Design review of the part built by this model. Coordinates are the model's own, in mm. Give positions to 0.01 mm unless a question says otherwise; leave off trailing zeros. Order: outer loops, then holes, each group sorted by start corner. A loop starts at its lowest first (then second) coordinate and runs counter-clockwise, first axis right, second up.
```python
from build123d import *

# Parameters (mm, degrees)
F0_W           = 127
F0_H           = 76.2
F1_DEPTH       = 3.175
F3_D           = 5.5
F3_CSINK_D     = 11.2
F3_CSINK_ANGLE = 90
F5_D           = 5.5
F5_CSINK_D     = 11.2
F5_CSINK_ANGLE = 90
F6_R           = 6.35


with BuildPart() as f1:
    # F0 (on Top) → F1 (new body)
    with BuildSketch(Plane.XY):
        Rectangle(F0_W, F0_H)
    extrude(amount=-F1_DEPTH)

    # F3 (through all)
    with Locations(Plane.XY):
        with Locations((-50.8, -25.4), (-50.8, 25.4), (50.8, 25.4), (50.8, -25.4)):
            CounterSinkHole(F3_D / 2, F3_CSINK_D / 2, counter_sink_angle=F3_CSINK_ANGLE)

    # F5 (through all)
    with Locations(Plane(origin=(0, 0, -3.175), x_dir=(1, 0, 0), z_dir=(0, 0, -1))):
        with Locations((0, 0)):
            CounterSinkHole(F5_D / 2, F5_CSINK_D / 2, counter_sink_angle=F5_CSINK_ANGLE)

    # F6
    f6_edges = [f1.edges().sort_by_distance(p)[0] for p in [
        (63.5, -38.1, -1.5875),
        (63.5, 38.1, -1.5875),
        (-63.5, -38.1, -1.5875),
        (-63.5, 38.1, -1.5875),
    ]]
    fillet(f6_edges, radius=F6_R)


solid = f1.part
```
1. For pin 1 (7 mm diameter, centred on x = 50.8, y = 25.4, fed in from -Z) (3 decimals); pin 2 (7 mm diameter, centred on x = 0, y = 0, fed in from -Z) (3 decimals); pin 3 (3.5 mm diameter, centred on x = -50.8, y = -25.4, fed in from +Z); pin 4 (6.5 mm diameter, centred on x = -50.8, y = 25.4, fed in from +Z), all flat-tipped, find the tip position at first contact; note any pin that passes through.
Recorded:
pin 1: stops at z = -3.175
pin 2: stops at z = -1.075
pin 3: passes through
pin 4: stops at z = -2.35
2. Take a section at C-C (z = -1.7). State the section outline as (x, y) points (3 decimals), then the cut area to 3 significant figures.
Recorded:
outline: (-63.5, -31.75) arc R6.35 ccw to (-57.15, -38.1) - (57.15, -38.1) arc R6.35 ccw to (63.5, -31.75) - (63.5, 31.75) arc R6.35 ccw to (57.15, 38.1) - (-57.15, 38.1) arc R6.35 ccw to (-63.5, 31.75) - close; hole circle Ø7.8 at (-50.8, -25.4); hole circle Ø7.8 at (-50.8, 25.4); hole circle Ø8.25 at (0, 0); hole circle Ø7.8 at (50.8, -25.4); hole circle Ø7.8 at (50.8, 25.4)
area: 9,400 mm2
3. Take a section at B-B (y = 25.4). State the section outline as (x, z) points (3 decimals), then the cut area to 3 significant figures.
Recorded:
outline: (-63.5, -3.175) - (-53.55, -3.175) - (-53.55, -2.85) - (-56.4, 0) - (-63.5, 0) - close; (-48.05, -3.175) - (48.05, -3.175) - (48.05, -2.85) - (45.2, 0) - (-45.2, 0) - (-48.05, -2.85) - close; (53.55, -3.175) - (63.5, -3.175) - (63.5, 0) - (56.4, 0) - (53.55, -2.85) - close
area: 352 mm2
4. Draft analysis for pull direction Y (two halves, no side actions). For faces 1 (the face through (-2.755, -0.868, -0.463)), 2 (the face through (63.5, 0, -2)), 3 (the face through (61.69, 36.19, -1.61)), state which applies: pulls with the +Y half, pulls with the -Y half, needs draft (parallel to the pull), parting line crosses it, or undercut.
Recorded:
face 1: undercut
face 2: needs draft
face 3: pulls with the +Y half
5. For line 1 along X through (y, z) = (-25.4, -2.95); line 2 along Y through (x, z) = (50.8, -3); line 3 along Y through (x, z) = (50, -0.3), list the stretches that pass through material, from the lowest coordinate up.
Recorded:
line 1: x = -63.5 to -53.55, -48.05 to 48.05, 53.55 to 63.5
line 2: y = -38.1 to -28.15, -22.65 to 22.65, 28.15 to 38.1
line 3: y = -38.1 to -30.64, -20.16 to 20.16, 30.64 to 38.1
6. Take a section at A-A (x = -50.8). State the section outline as (y, z) points (3 decimals).
Recorded:
outline: (-38.1, -3.175) - (-28.15, -3.175) - (-28.15, -2.85) - (-31, 0) - (-38.1, 0) - close; (-22.65, -3.175) - (22.65, -3.175) - (22.65, -2.85) - (19.8, 0) - (-19.8, 0) - (-22.65, -2.85) - close; (28.15, -3.175) - (38.1, -3.175) - (38.1, 0) - (31, 0) - (28.15, -2.85) - close
7. Take a section at D-D (y = 0). State the section outline as (x, z) points (3 decimals).
Recorded:
outline: (-63.5, -3.175) - (-5.6, -3.175) - (-2.75, -0.325) - (-2.75, 0) - (-63.5, 0) - close; (2.75, -0.325) - (5.6, -3.175) - (63.5, -3.175) - (63.5, 0) - (2.75, 0) - close
